Check sheet for the drawn part. Datum: minimum x, y, z corner. Units: mm. Give positions to 0.01 mm unless a question says otherwise; leave off trailing zeros. Loops run counter-clockwise (first coordinate to the right, second up) from the corner with the lowest first, then second, coordinate; pieces in that order, holes last. Notation, with made-up numbers: (44, 45.25) - (100, 45.25) arc R27 cw to (100, 82.25) - close; hole circle Ø5 at (87, -24). An arc over 180 degrees is marked (long way). Use a Markdown table: item, result. Add a question column.
1. Depth check by flat-ended pin: P1, Ø3, axis at x = 5, y = 66, coming from the -Z side. Enter the tip coordinate at first touch or a pass-through.
2. Material ranges on L1, parallel to Y at x = 5, z = 2.7; L2, parallel to X at y = 6, z = 0.5, recorded low to high.
3. Cross-section at A-A on y = 35.5. Enter the section's corners in (x, z), and give its area (3 significant figures).
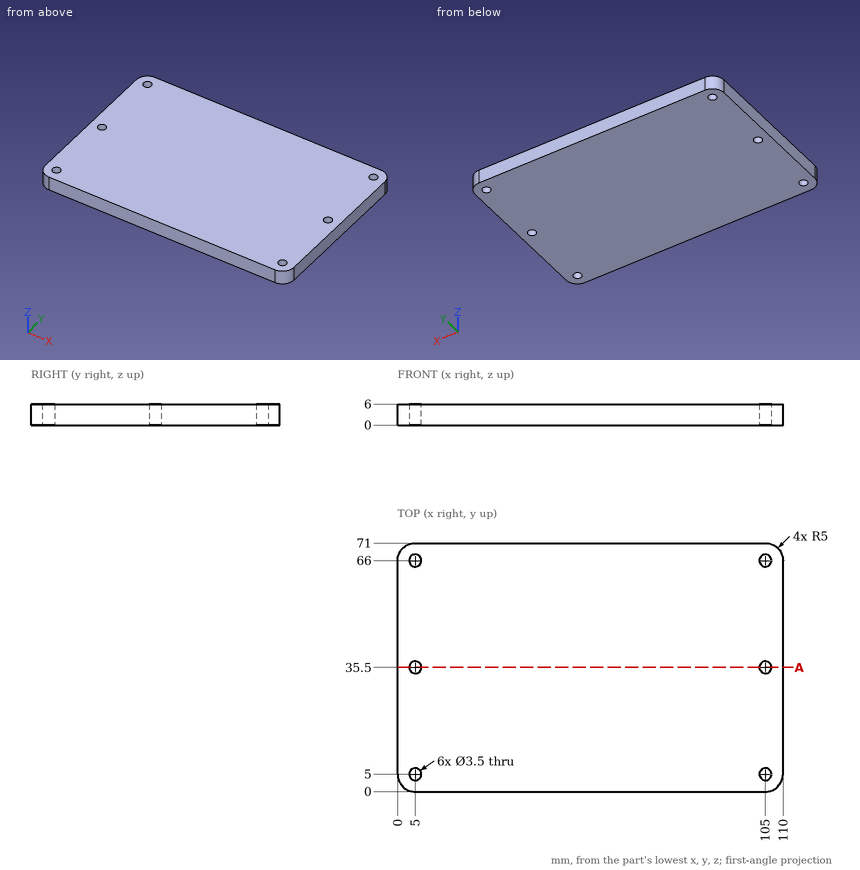
Values found:
| question | item | result |
|---|---|---|
| 1 | P1 | passes through |
| 2 | L1 | y = 0 to 3.25, 6.75 to 33.75, 37.25 to 64.25, 67.75 to 71 |
| 2 | L2 | x = 0 to 3.56, 6.44 to 103.56, 106.44 to 110 |
| 3 | outline | (0, 0) - (3.25, 0) - (3.25, 6) - (0, 6) - close; (6.75, 0) - (103.25, 0) - (103.25, 6) - (6.75, 6) - close; (106.75, 0) - (110, 0) - (110, 6) - (106.75, 6) - close |
| 3 | area | 618 mm2 |
